The listing builds one solid part. Answer for the finished solid, in the listing's coordinates (mm). A direction names the side the tool comes from. Coordinates: 2 decimals unless noted, no trailing zeros. Loops run counter-clockwise (first coordinate to the right, second up) from the corner with the lowest first, then second, coordinate; pieces in that order, holes last. Notation, with made-up numbers: (67, 47.5) - (78, 47.5) arc R12 cw to (78, 68.5) - close; hole circle Ø9 at (86, 89). An arc over 180 degrees is marked (long way). Use one line per item in the form item = value. Start each with the question number.
```python
from build123d import *

# Parameters (mm, degrees)
F0_W     = 123.2712268829
F0_H     = 69.5435777307
F1_DEPTH = 25.4
F2_W     = 123.2712268829
F2_H     = 4.1865706444
F2_H_2   = 5.5820941925
F3_DEPTH = 19.05
F4_W     = 58.4956854582
F4_H     = 59.7749128938
F5_DEPTH = 19.05
F6_R     = 7.8204757045
F7_DEPTH = 84.836
F8_R     = 7.993016925
F9_DEPTH = 31.242


with BuildPart() as f1:
    # F0 (on Front) → F1 (new body)
    with BuildSketch(Plane.XZ):
        with Locations((3.1399279833, -2.4421662092)):
            Rectangle(F0_W, F0_H)
    extrude(amount=F1_DEPTH)

    # F2 (on face) → F3 (cut)
    with BuildSketch(Plane.XZ.offset(25.4)):
        with Locations((3.1399279833, 30.2363373339)):
            Rectangle(F2_W, F2_H)
        with Locations((3.1399279833, -34.4229079783)):
            Rectangle(F2_W, F2_H_2)
    extrude(amount=-F3_DEPTH, mode=Mode.SUBTRACT)

    # F4 (on face) → F5 (join)
    with BuildSketch(Plane.XZ.offset(25.4)):
        with Locations((-29.2478427291, -1.7444044352)):
            Rectangle(F4_W, F4_H)
    extrude(amount=F5_DEPTH)

    # F6 (on face) → F7 (cut)
    with BuildSketch(Plane.XZ.offset(44.45)):
        with Locations((-29.2478427291, 0)):
            Circle(F6_R)
    extrude(amount=-F7_DEPTH, mode=Mode.SUBTRACT)

    # F8 (on face) → F9 (cut)
    with BuildSketch(Plane.XZ.offset(25.4)):
        with Locations((33.1436805427, 0)):
            Circle(F8_R)
    extrude(amount=-F9_DEPTH, mode=Mode.SUBTRACT)


solid = f1.part
```
(1) A cutting plane is placed at A-A (z = 0). Determine the outline of the cut face in (x, y), then the cut area to 3 significant figures.
(2) A cutting plane is placed at C-C (x = 5). Determine the outline of the cut face in (y, z), then the cut area to 3 significant figures.
(3) Each of these flat-tipped pins is pushed along its axis until it touches: pin 1 Ø6 at (x, z) = (-39, 22) entering from +Y; pin 2 Ø3 at (x, z) = (35, 15) entering from -Y; pin 3 Ø5.5 at (y, z) = (-32, -8) entering from +X; pin 4 Ø3.5 at (x, z) = (-20.5, 31) entering from -Y. Where does it stop, or does it pass through?
(4) For faces 1 (the face through (25, -25.4, -1)), 2 (the face through (-11, -21, 28.143)), 3 (the face through (-11, -21, -31.632)), determine the directions among +Z, -Z, +X, -X, +Y, -Y from which every point of the face is accessible in a straight line to the end or side of a thin tool.
(5) A cutting plane is placed at D-D (y = -36). Determine the outline of the cut face in (x, z).
(6) A cutting plane is placed at B-B (y = -15). Determine the outline of the cut face in (x, z), then the cut area to 3 significant figures.
(7) Find the intervals of material crossed by probe 1 along X at (y, z) = (-20.5, -7); probe 2 along Z at (x, y) = (-6, -26); probe 3 along Y at (x, z) = (48, -24), in increasing order. Write a range as from..to.
(8) Determine the mould class of faces 4 (the face through (2, -6.35, -34)), 5 (the face through (-25.64, -22.54, -6.94)), 6 (the face through (0, -35, -2)) for opening direction X: +X half, -X half, draft (parallel to the pull), parting line (faces both ways), or undercut.
Evaluation:
q1.outline = (-58.5, -44.45) - (-37.07, -44.45) - (-37.07, 0) - (-58.5, 0) - close; (-21.43, -44.45) - (0, -44.45) - (0, -25.4) - (25.15, -25.4) - (25.15, 0) - (-21.43, 0) - close; (41.14, -25.4) - (64.78, -25.4) - (64.78, 0) - (41.14, 0) - close
q1.area = 3,140 mm^2
q2.outline = (-25.4, -31.63) - (-6.35, -31.63) - (-6.35, -37.21) - (0, -37.21) - (0, 32.33) - (-6.35, 32.33) - (-6.35, 28.14) - (-25.4, 28.14) - close
q2.area = 1,580 mm^2
q3.pin_1 = 0
q3.pin_2 = -25.4
q3.pin_3 = 0
q3.pin_4 = -6.35
q4.face_1 = +Z, -Z, +X, -Y
q4.face_2 = +Z, +X, -X, -Y
q4.face_3 = -Z, +X, -X, -Y
q5.outline = (-58.5, -31.63) - (0, -31.63) - (0, 28.14) - (-58.5, 28.14) - close; hole circle Ø15.64 at (-29.25, 0)
q6.outline = (-58.5, -31.63) - (64.78, -31.63) - (64.78, 28.14) - (-58.5, 28.14) - close; hole circle Ø15.64 at (-29.25, 0); hole circle Ø15.99 at (33.14, 0)
q6.area = 6,980 mm^2
q7.probe_1 = -58.5..-32.73, -25.76..29.29, 37..64.78
q7.probe_2 = -31.63..28.14
q7.probe_3 = -25.4..0
q8.face_4 = draft
q8.face_5 = undercut
q8.face_6 = +X half
